Could you check a few things on this model? Use its own coordinates, in mm. A direction names the side the tool comes from. Give positions to 0.01 mm unless a question says otherwise; leave off trailing zeros. Write each loop counter-clockwise with the first axis right and the second up, starting at its lowest first coordinate (ties: lowest second). Pieces come first, ordered by that corner, then holes. Notation, with made-up numbers: M 87.25,58.5 L 135.25,58.5 A17 cw 135.25,67.5 Z; hole C -15,5 d5. An arc over 180 degrees is marked long. Write each question's results on one line, items separated by ' | '. Start each with the question number.
from build123d import *

# Parameters (mm, degrees)
F0_W     = 53.34
F0_H     = 69.102946
F1_DEPTH = 6.35
F3_DEPTH = 25.4
F4_W     = 6.35
F4_H     = 38.1
F5_DEPTH = 63.5
F6_R     = 12.7
F7_DEPTH = 53.34
F8_R     = 10.16
F9_DEPTH = 53.34


with BuildPart() as f1:
    # F0 (on Front) → F1 (new body, symmetric)
    with BuildSketch(Plane.XZ):
        with BuildLine():
            Line((26.67, 37.667938), (13.800602, 62.397646))
            ThreePointArc((13.800602, 62.397646), (0, 70.77328), (-13.800602, 62.397646))
            Line((-13.800602, 62.397646), (-26.67, 37.667938))
            Line((-26.67, 37.667938), (-26.67, 30.885875))
            Line((-26.67, 30.885875), (26.67, 30.885875))
            Line((26.67, 30.885875), (26.67, 37.667938))
        make_face()
        with Locations((0, -3.665598)):
            Rectangle(F0_W, F0_H)
    extrude(amount=F1_DEPTH, both=True)

    # F2 (on face) → F3 (cut)
    with BuildSketch(Plane(origin=(0, 6.35, 0), x_dir=(-1, 0, 0), z_dir=(0, 1, 0))):
        Polygon((-23.622, 31.317938), (-23.622, -38.217071), (23.622, -38.217071), (23.622, 31.317938), (18.919615, 31.317938), (18.919615, 37.667938), (-16.959142, 37.667938), (-16.959142, 31.317938), align=None)
    extrude(amount=-F3_DEPTH, mode=Mode.SUBTRACT)

    # F4 (on face) → F5 (cut)
    with BuildSketch(Plane.YZ.offset(26.67)):
        with Locations((-3.175, 56.717938)):
            Rectangle(F4_W, F4_H)
    extrude(amount=-F5_DEPTH, mode=Mode.SUBTRACT)

    # F6 (on face) → F7 (join)
    with BuildSketch(Plane.YZ.offset(26.67)):
        with Locations((0, -49.258824)):
            Circle(F6_R)
    extrude(amount=-F7_DEPTH)

    # F8 (on face) → F9 (cut)
    with BuildSketch(Plane.YZ.offset(26.67)):
        with Locations((0, -49.258824)):
            Circle(F8_R)
    extrude(amount=-F9_DEPTH, mode=Mode.SUBTRACT)


solid = f1.part
Q1. If we section it at C-C (y = 2.5): Please give me the cut outline in (x, z) (1 decimal).
Q2. If we section it at B-B (x = 20): Please give me the cut outline in (y, z).
Q3. Please list where these lines run through material, in increasing order: line 1 (X direction, y = 0, z = 7); line 2 (Z direction, x = 22.5, y = 2); line 3 (Y direction, x = -24, z = -12.5). Write a range as [from, to].
Q4. If we section it at A-A (z = -11): Please give me the cut outline in (x, y).
Q5. I'm going to push flat-ended pins straight in: P1, Ø3, axis at x = -19, y = -0.5, coming from the +Z side; P2, Ø1.9, axis at x = -21.5, y = -1.5, coming from the +Z side; P3, Ø12, axis at x = -12.5, y = -9.5, coming from the +Z side. Where does each tip first touch, or does it pass through?
Q6. If we mould it in two halves opening along X, with no side actions, what happens to faces 5 (the face through (-21, 0, 31.318)), 6 (the face through (26.67, 0, 0)), 7 (the face through (-25, -6.35, 0)), 8 (the face through (16.959, 0, 35))? For each: pulls with the +X half, pulls with the -X half, needs draft (parallel to the pull), parting line crosses it, or undercut.
Q7. If we section it at D-D (y = -8.25): Please give me the cut outline in (x, z).
Q8. For faces 1 (the face through (22, -3, 37.668)), 2 (the face through (-1, 3, 37.668)), 3 (the face through (0.373, -2.202, -59.177)), 4 (the face through (-2, 6.35, 41)), which set-ups out of +Z, -Z, +X, -X, +Y, -Y let a thin tool reach every point of the face, with its end or its side?
Determined:
1) outline: M -26.7,-61.7 L 26.7,-61.7 L 26.7,-59.1 L -26.7,-59.1 Z; M -26.7,-39.4 L 26.7,-39.4 L 26.7,37.7 L 13.8,62.4 A15.6 ccw -13.8,62.4 L -26.7,37.7 Z; hole M -23.6,-36.8 L 23.6,-36.8 L 23.6,31.3 L 17,31.3 L 17,37.7 L -18.9,37.7 L -18.9,31.3 L -23.6,31.3 Z
2) outline: C 0,-49.26 d25.4; M -6.35,31.32 L 6.35,31.32 L 6.35,50.48 L 0,50.48 L 0,37.67 L -6.35,37.67 Z; hole C 0,-49.26 d20.32
3) line 1: x = [-26.67, -23.62], [23.62, 26.67] | line 2: z = [-61.8, -59.22], [-39.3, -36.72], [31.32, 45.68] | line 3: y = [-6.35, 6.35]
4) outline: M -26.67,-6.35 L -23.62,-6.35 L -23.62,6.35 L -26.67,6.35 Z; M 23.62,-6.35 L 26.67,-6.35 L 26.67,6.35 L 23.62,6.35 Z
5) P1: stops at z = 55.12 | P2: stops at z = 37.67 | P3: stops at z = -37.05
6) face 5: undercut | face 6: pulls with the +X half | face 7: needs draft | face 8: undercut
7) outline: M -26.67,-58.91 L 26.67,-58.91 L 26.67,-55.19 L -26.67,-55.19 Z; M -26.67,-43.33 L 26.67,-43.33 L 26.67,-39.6 L -26.67,-39.6 Z
8) face 1: +Z, +X, -X, -Y | face 2: +Y, -Y | face 3: +X, -X | face 4: +Z, +X, -X, +Y
